from build123d import *

# Parameters (mm, degrees)
F1_DEPTH = 25.4
F2_R     = 6.35
F3_DEPTH = 25.4


with BuildPart() as f1:
    # F0 (on Front) → F1 (new body)
    with BuildSketch(Plane.XZ):
        Polygon((0, 12.7), (0, 0), (76.2, 0), (76.2, 12.7), (50.8, 12.7), (50.8, 44.45), (25.4, 44.45), (25.4, 12.7), align=None)
    extrude(amount=F1_DEPTH)

    # F2 (on face) → F3 (cut)
    with BuildSketch(Plane.YZ.offset(50.8)):
        with BuildLine():
            ThreePointArc((-9.5586421261, 44.45), (-2.7865480563, 40.0861130576), (0, 32.5270180545))
            Line((0, 32.5270180545), (0, 44.45))
            Line((0, 44.45), (-9.5586421261, 44.45))
        make_face()
        with BuildLine():
            ThreePointArc((-25.4, 32.5270180545), (-22.6134519437, 40.0861130576), (-15.8413578739, 44.45))
            Line((-15.8413578739, 44.45), (-25.4, 44.45))
            Line((-25.4, 44.45), (-25.4, 32.5270180545))
        make_face()
        with Locations((-12.7, 31.75)):
            Circle(F2_R)
    extrude(amount=-F3_DEPTH, mode=Mode.SUBTRACT)


solid = f1.part
Source: CAD feature listing. Evaluate the final solid. Frame: model axes, mm. A direction names the side the tool comes from. Coordinates: 2 decimals unless noted, no trailing zeros. Loops run counter-clockwise (first coordinate to the right, second up) from the corner with the lowest first, then second, coordinate; pieces in that order, holes last. Notation, with made-up numbers: (-36.75, 42.5) - (11.25, 42.5) arc R7 ccw to (11.25, 46.5) - close; hole circle Ø3 at (70.5, 73.5). An arc over 180 degrees is marked (long way). One line per item, written item: value. Start each with the question number.
1. Section D-D (z = 16). Return the cut outline in (x, y).
2. Mould query, pull axis Z, two halves, no side actions, for faces 1 (the flat face through (76.2, -13, 6)), 2 (the cylindrical face through (38.278, -6.643, 33.657)), 3 (the cylindrical face through (38.28, -22.68, 40)). Classes: pulls with the +Z half, pulls with the -Z half, needs draft (parallel to the pull), parting line crosses it, or undercut.
3. Set-up query: faces 4 (the flat face through (13, -13, 12.7)), 5 (the flat face through (38, -13, 0)), 6 (the flat face through (50.8, -13, 25)). Return all of +Z, -Z, +X, -X, +Y, -Y with unobstructed straight access to the full face (end or side cutting, diameter ignored); none if empty.
4. Section A-A (z = 31.75). Return the cut outline in (x, y).
5. Section C-C (x = 35). Return the cut outline in (y, z).
6. Contact query for flat-ended pins moving along their axis: P1, Ø7.5, axis at y = -12.7, z = 31.75, coming from the +X side; P2, Ø12.5, axis at y = -16, z = 31.5, coming from the -X side; P3, Ø12, axis at x = 64, y = -13, coming from the +Z side. Output: stop coordinate, or through.
7. Ray query, L1, parallel to Z at x = 43.5, y = -12.7; L2, parallel to Z at x = 68, y = -23; L3, parallel to Y at x = 43.5, z = 26. Return the intervals inside material, ascending.
8. Section B-B (y = -12.7). Return the cut outline in (x, z), and give its area (3 significant figures).
Verdict:
1. outline: (25.4, -25.4) - (50.8, -25.4) - (50.8, 0) - (25.4, 0) - close
2. face 1: needs draft
2. face 2: undercut
2. face 3: pulls with the +Z half
3. face 4: +Z, -X, +Y, -Y
3. face 5: -Z, +X, -X, +Y, -Y
3. face 6: +Z, +X, +Y, -Y
4. outline: (25.4, -25.4) - (50.8, -25.4) - (50.8, -19.05) - (25.4, -19.05) - close; (25.4, -6.35) - (50.8, -6.35) - (50.8, 0) - (25.4, 0) - close
5. outline: (-25.4, 0) - (0, 0) - (0, 32.53) arc R12.71 ccw to (-9.56, 44.45) - (-15.84, 44.45) arc R12.71 ccw to (-25.4, 32.53) - close; hole circle Ø12.7 at (-12.7, 31.75)
6. P1: passes through
6. P2: stops at x = 25.4
6. P3: stops at z = 12.7
7. L1: z = 0 to 25.4, 38.1 to 44.45
7. L2: z = 0 to 12.7
7. L3: y = -25.4 to -15.39, -10.01 to 0
8. outline: (0, 0) - (76.2, 0) - (76.2, 12.7) - (50.8, 12.7) - (50.8, 25.4) - (25.4, 25.4) - (25.4, 12.7) - (0, 12.7) - close; (25.4, 38.1) - (50.8, 38.1) - (50.8, 44.45) - (25.4, 44.45) - close
8. area: 1,450 mm2
